Part print with two shaded views. Sizes in mm from the minimum x, y, z corner. A direction names the side the tool comes from. Round coordinates to 2 decimals unless told otherwise and drop trailing zeros. Write each loop counter-clockwise with the first axis right and the second up, starting at its lowest first coordinate (ties: lowest second). Pieces come first, ordered by that corner, then holes. Notation, with made-up numbers: (-16, -21.75) -> (-12, -21.75) arc R25 cw to (-12, 0.25) -> close; hole circle Ø2 at (13, -15). An arc over 180 degrees is marked (long way). Answer as CSV lines item,"result".
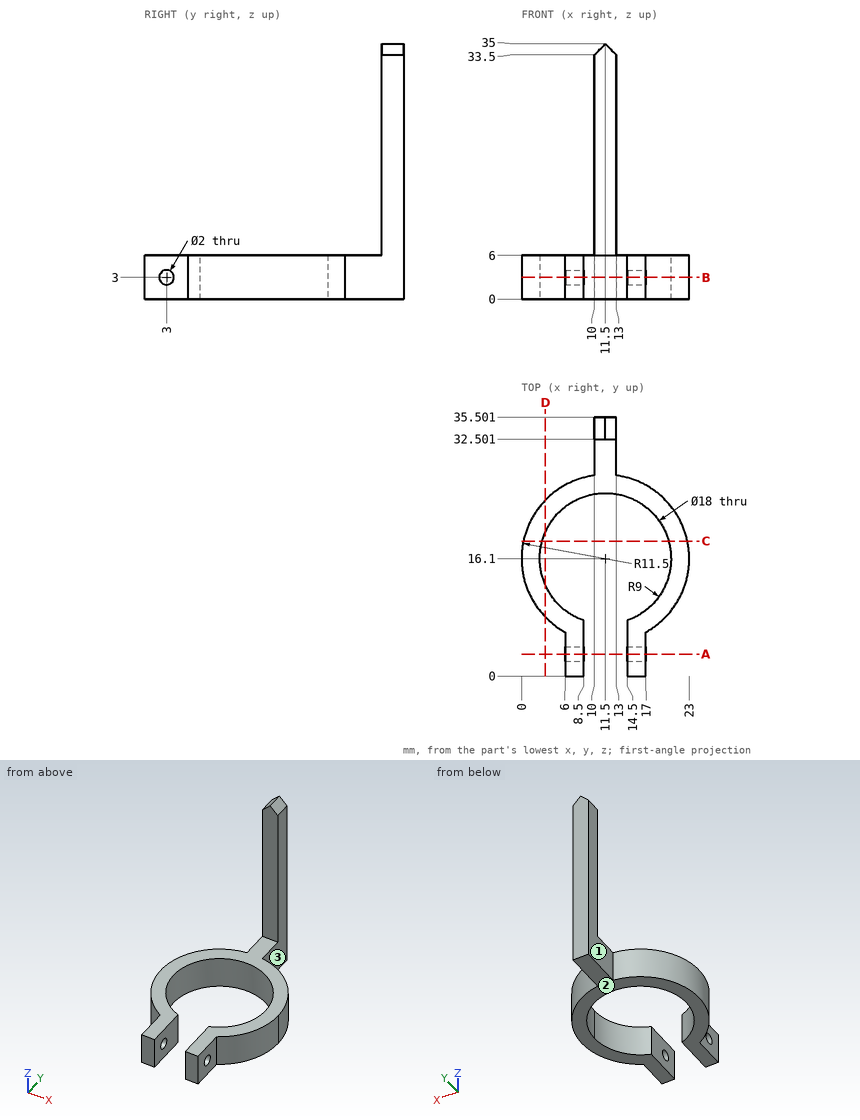
1. Cut at A-A, the plane y = 3. Write the cut outline in (x, z).
Results found:
outline,"(6, 0) -> (8.5, 0) -> (8.5, 2) -> (6, 2) -> close; (6, 4) -> (8.5, 4) -> (8.5, 6) -> (6, 6) -> close; (14.5, 0) -> (17, 0) -> (17, 2) -> (14.5, 2) -> close; (14.5, 4) -> (17, 4) -> (17, 6) -> (14.5, 6) -> close"
2. Drop flat-ended pins along their axis: pin 1 Ø4 at (x, z) = (17, 8.5) entering from -Y; pin 2 Ø1.8 at (y, z) = (3.5, 4) entering from +X; pin 3 Ø1.8 at (y, z) = (4.5, 2.5) entering from -X; pin 4 Ø6.5 at (y, z) = (31, 14) entering from +X. Give the stop position or say it passes through.
Results found:
pin 1,"passes through"
pin 2,"stops at x = 17"
pin 3,"stops at x = 6"
pin 4,"stops at x = 13"
3. Cut at B-B, the plane z = 3. Write the cut outline in (x, y) (1 decimal).
Results found:
outline,"(6, 0) -> (8.5, 0) -> (8.5, 2) -> (6, 2) -> close; (6, 4) -> (8.5, 4) -> (8.5, 7.6) arc R9 cw (long way) to (14.5, 7.6) -> (14.5, 4) -> (17, 4) -> (17, 6) arc R11.5 ccw to (13, 27.5) -> (13, 35.5) -> (10, 35.5) -> (10, 27.5) arc R11.5 ccw to (6, 6) -> close; (14.5, 0) -> (17, 0) -> (17, 2) -> (14.5, 2) -> close"
4. Cut at D-D, the plane x = 3.25. Write the cut outline in (y, z).
Results found:
outline,"(8.09, 0) -> (12.5, 0) -> (12.5, 6) -> (8.09, 6) -> close; (19.7, 0) -> (24.11, 0) -> (24.11, 6) -> (19.7, 6) -> close"
5. Cut at C-C, the plane y = 18.5. Write the cut outline in (x, z).
Results found:
outline,"(0.25, 0) -> (2.83, 0) -> (2.83, 6) -> (0.25, 6) -> close; (20.17, 0) -> (22.75, 0) -> (22.75, 6) -> (20.17, 6) -> close"
6. Which spindle directions (+Z, -Z, +X, -X, +Y, -Y) get a long thin tool onto all of the face, cutting with end or side? Do the marked faces 1, 2 and 3. Say none if no direction does.
Results found:
face 1,"+Z, -Z, -X, +Y"
face 2,"-Z, +X, -X, +Y, -Y"
face 3,"+Z, -Z, +X, +Y"
7. Probe line 1 along Z through (x, y) = (6.9, 3); line 2 along Y through (x, z) = (12.5, 29); line 3 along Z through (x, y) = (21.25, 12.5). List the from-to ranges inside material, lowest first.
Results found:
line 1,"z = 0 to 2, 4 to 6"
line 2,"y = 32.5 to 35.5"
line 3,"z = 0 to 6"
